```python
from build123d import *

# Parameters (mm, degrees)
ESQUISSE3_R             = 2.35
BOSS_EXTRU_2_DEPTH      = 70.2
CHANFREIN1_SIZE         = 5
ESQUISSE6_R             = 3.2
ESQUISSE6_R_2           = 2.35
ENL_V_MAT_EXTRU_1_DEPTH = 7
ENL_V_START             = -7
ESQUISSE7_R             = 3.2
ESQUISSE7_R_2           = 2.35
ENL_V_MAT_EXTRU_2_DEPTH = 7
ENL_V_MAT_EXTRU_4_DEPTH = 2


with BuildPart() as part:
    # Esquisse3 → Boss.-Extru.2 (new, symmetric)
    with BuildSketch(Plane(origin=(0, 0, 0), x_dir=(0, 0, -1), z_dir=(1, 0, 0))):
        Polygon((-4.5, -10.5), (-4.5, 4.5), (10.5, 4.5), (10.5, -4.5), (4.5, -4.5), (4.5, -10.5), align=None)
        with Locations((1.5, -1.5)):
            Circle(ESQUISSE3_R, mode=Mode.SUBTRACT)
    extrude(amount=BOSS_EXTRU_2_DEPTH, both=True)

    # Chanfrein1
    chanfrein1_edges = [part.edges().sort_by_distance(p)[0] for p in [
        (0, 4.5, 4.5),
    ]]
    chamfer(chanfrein1_edges, length=CHANFREIN1_SIZE)

    # Esquisse6 → Enlèv. mat.-Extru.1 (cut)
    with BuildSketch(Plane.ZY.offset(70.2)):
        with Locations((-1.5, -1.5)):
            Circle(ESQUISSE6_R)
        with Locations((-1.5, -1.5)):
            Circle(ESQUISSE6_R_2, mode=Mode.SUBTRACT)
    extrude(amount=-ENL_V_MAT_EXTRU_1_DEPTH, mode=Mode.SUBTRACT)

    # Esquisse7 → Enlèv. mat.-Extru.2 (cut)
    with BuildSketch(Plane(origin=(70.2, 0, 0), x_dir=(0, 0, -1), z_dir=(1, 0, 0)).offset(ENL_V_START)):
        with Locations(Location((1.5, -1.5, 0), (0, 0, 180))):
            Circle(ESQUISSE7_R)
        with Locations(Location((1.5, -1.5, 0), (0, 0, 180))):
            Circle(ESQUISSE7_R_2, mode=Mode.SUBTRACT)
    extrude(amount=ENL_V_MAT_EXTRU_2_DEPTH, mode=Mode.SUBTRACT)

    # Esquisse9 → Enlèv. mat.-Extru.4 (cut)
    with BuildSketch(Plane.XY.offset(4.5)):
        with BuildLine():
            Line((-48.7, -1.3), (-41.7, -1.3))
            ThreePointArc((-41.7, -1.3), (-37.5, -5.5), (-41.7, -9.7))
            Line((-41.7, -9.7), (-48.7, -9.7))
            ThreePointArc((-48.7, -9.7), (-52.9, -5.5), (-48.7, -1.3))
        make_face()
    extrude(amount=-ENL_V_MAT_EXTRU_4_DEPTH, mode=Mode.SUBTRACT)


solid = part.part
```
The model under review builds one solid part; all positions refer to its coordinate system, in mm. A direction names the side the tool comes from. Coordinates: 2 decimals unless noted, no trailing zeros. Order: outer loops, then holes, each group sorted by start corner. A loop starts at its lowest first (then second) coordinate and runs counter-clockwise, first axis right, second up. Notation, with made-up numbers: (-4, -18) -> (42, -18) arc R17 cw to (42, -8) -> close; hole circle Ø3 at (49, 46). An arc over 180 degrees is marked (long way). Answer in a Markdown table with one row per item. Add a question column.
Item 1: We need section A-A on x = -6.5. Write out the cut boundary in (y, z).
Item 2: We need section B-B on y = -6.25. Write out the cut boundary in (x, z), plus the area to 3 significant figures.
Item 3: Machinability: for faces 1 (the cylindrical face through (-52.9, -5.6, 3.5)), 2 (the cylindrical face through (66.651, -0.274, 1.456)), 3 (the flat face through (1, -7, -4.5)), 4 (the cylindrical face through (-66.749, -0.539, 1.552)), 5 (the flat face through (1, -6, 4.5)), which of the approach directions +Z, -Z, +X, -X, +Y, -Y give a long, thin tool a straight path to every point of the face, cutting with its end or side? Answer none if there is none.
Item 4: Mouldability with a two-part tool opening along X and no side actions: class faces 6 (the flat face through (-63.2, 1, -2)), 7 (the flat face through (-45, -5, 2.5)), 8 (the flat face through (63.2, -4, -2)), 9 (the flat face through (1, -4.5, -8)) as +X half, -X half, draft (parallel to the pull), parting line (faces both ways), or undercut.
Item 5: Clearance check with flat-ended pins moving along their axes: pin 1 (8 mm diameter, centred on y = -1, z = -2.5, fed in from -X); pin 2 (3 mm diameter, centred on x = 29.5, y = -6.5, fed in from -Z); pin 3 (1.5 mm diameter, centred on x = 5.5, z = 0.5, fed in from +Y); pin 4 (6 mm diameter, centred on y = -1.5, z = -1.5, fed in from +X). State where each tip first meets the part, or that it passes through.
Item 6: To check wall thickness, follow probe 1 along Y at (x, z) = (65.75, -1.5); probe 2 along Y at (x, z) = (31.5, -1.5); probe 3 along Y at (x, z) = (-35.5, -7.75). State the ranges of each line that lie inside material, in increasing order.
Item 7: We need section C-C on x = -40. Write out the cut boundary in (y, z), plus the area to 3 significant figures.
Item 8: We need section D-D on z = -8.5. Write out the cut boundary in (x, y).
Final values:
| question | item | result |
|---|---|---|
| 1 | outline | (-10.5, -4.5) -> (-4.5, -4.5) -> (-4.5, -10.5) -> (4.5, -10.5) -> (4.5, -0.5) -> (-0.5, 4.5) -> (-10.5, 4.5) -> close; hole circle Ø4.7 at (-1.5, -1.5) |
| 2 | outline | (-70.2, -4.5) -> (70.2, -4.5) -> (70.2, 4.5) -> (-37.57, 4.5) -> (-37.57, 2.5) -> (-52.83, 2.5) -> (-52.83, 4.5) -> (-70.2, 4.5) -> close |
| 2 | area | 1,230 mm2 |
| 3 | face 1 | +Z |
| 3 | face 2 | +X |
| 3 | face 3 | -Z, +X, -X, -Y |
| 3 | face 4 | -X |
| 3 | face 5 | +Z, +X, -X, +Y, -Y |
| 4 | face 6 | -X half |
| 4 | face 7 | undercut |
| 4 | face 8 | +X half |
| 4 | face 9 | draft |
| 5 | pin 1 | stops at x = -70.2 |
| 5 | pin 2 | stops at z = -4.5 |
| 5 | pin 3 | stops at y = 4.25 |
| 5 | pin 4 | stops at x = 63.2 |
| 6 | probe 1 | y = -10.5 to -4.7, 1.7 to 4.5 |
| 6 | probe 2 | y = -10.5 to -3.85, 0.85 to 4.5 |
| 6 | probe 3 | y = -4.5 to 4.5 |
| 7 | outline | (-10.5, -4.5) -> (-4.5, -4.5) -> (-4.5, -10.5) -> (4.5, -10.5) -> (4.5, -0.5) -> (-0.5, 4.5) -> (-1.66, 4.5) -> (-1.66, 2.5) -> (-9.34, 2.5) -> (-9.34, 4.5) -> (-10.5, 4.5) -> close; hole circle Ø4.7 at (-1.5, -1.5) |
| 7 | area | 144 mm2 |
| 8 | outline | (-70.2, -4.5) -> (70.2, -4.5) -> (70.2, 4.5) -> (-70.2, 4.5) -> close |
